Input: part model. Units: mm. Frame: model coordinates. A direction names the side the tool comes from. Give positions to 0.01 mm unless a question says otherwise; leave off trailing zeros. Write each loop counter-clockwise with the first axis right and the second up, starting at its lowest first coordinate (ties: lowest second). Pieces come first, ordered by that corner, then holes. Notation, with made-up numbers: (88.5, 43.5) -> (126.5, 43.5) arc R35 ccw to (126.5, 75.5) -> close; hole circle Ø11 at (22, 50.25). An arc over 180 degrees is marked (long way). Return JSON: item names as keys, results as strings. Group by question number.
Item 1: Section C-C, the plane y = 13. Return loops of the section in (x, z) (3 decimals), then the cut area to 3 significant figures.
Item 2: Section B-B, the plane x = 0. Return loops of the section in (y, z) (3 decimals).
Item 3: Mould query, pull axis Y, two halves, no side actions, for faces 3 (the face through (38.1, -1.5, 3.9)), 4 (the face through (27.746, 10.498, -23.835)), 5 (the face through (-1, -3.175, 7)). Classes: released by +Y, released by -Y, zero draft, split by the parting line, or undercut.
Item 4: Section A-A, the plane x = 25.4. Return loops of the section in (y, z) (3 decimals).
Item 5: Set-up query: faces 1 (the face through (-27.332, -1.565, 27.025)), 2 (the face through (-1, 0, 8)). Return all of +Z, -Z, +X, -X, +Y, -Y with unobstructed straight access to the full face (end or side cutting, diameter ignored); none if empty.
Item 6: Section D-D, the plane z = 6. Return loops of the section in (x, y) (3 decimals), then the cut area to 3 significant figures.
Item 7: Pin query (flat end, axial travel): P1, Ø6, axis at x = 0, z = -3.175, coming from the -Y side; P2, Ø6, axis at x = -21.5, z = 19.5, coming from the +Y side. Return the tip coordinate at first contact, or that it passes through.
Item 8: Line query: line 1 (Z direction, x = 19, y = -1); line 2 (Y direction, x = 25.4, z = -23.85) (3 decimals); line 3 (Y direction, x = -27.5, z = 11) (3 decimals). Output: solid intervals per line, ascending. Write a range as [from, to].
from build123d import *

# Parameters (mm, degrees)
F0_W     = 76.2
F0_H     = 63.5
F0_R     = 1.5875
F0_R_2   = 3.81
F1_DEPTH = 3.175
F3_W     = 76.2
F3_H     = 19.05
F3_R     = 2.54
F4_DEPTH = 3.175
F5_R     = 1.27


with BuildPart() as f1:
    # F0 (on Front) → F1 (new body)
    with BuildSketch(Plane.XZ):
        with Locations((0, 6.35)):
            Rectangle(F0_W, F0_H)
        with Locations((-26.9875, -3.175)):
            Circle(F0_R, mode=Mode.SUBTRACT)
        with Locations((-19.05, -3.175)):
            Circle(F0_R_2, mode=Mode.SUBTRACT)
        with Locations((-7.9375, -3.175)):
            Circle(F0_R, mode=Mode.SUBTRACT)
        with Locations((0, -3.175)):
            Circle(F0_R_2, mode=Mode.SUBTRACT)
        with Locations((11.1125, -3.175)):
            Circle(F0_R, mode=Mode.SUBTRACT)
        with Locations((19.05, -3.175)):
            Circle(F0_R_2, mode=Mode.SUBTRACT)
        with Locations((-26.9875, 28.575)):
            Circle(F0_R, mode=Mode.SUBTRACT)
        with Locations((-19.05, 28.575)):
            Circle(F0_R_2, mode=Mode.SUBTRACT)
        with Locations((-7.9375, 28.575)):
            Circle(F0_R, mode=Mode.SUBTRACT)
        with Locations((0, 28.575)):
            Circle(F0_R_2, mode=Mode.SUBTRACT)
        with Locations((11.1125, 28.575)):
            Circle(F0_R, mode=Mode.SUBTRACT)
        with Locations((19.05, 28.575)):
            Circle(F0_R_2, mode=Mode.SUBTRACT)
    extrude(amount=F1_DEPTH)

    # F3 (on face) → F4 (join)
    with BuildSketch(Plane(origin=(0, 0, -25.4), x_dir=(1, 0, 0), z_dir=(0, 0, -1))):
        with Locations((0, -9.525)):
            Rectangle(F3_W, F3_H)
        with Locations((-25.4, -9.525)):
            Circle(F3_R, mode=Mode.SUBTRACT)
        with Locations((25.4, -9.525)):
            Circle(F3_R, mode=Mode.SUBTRACT)
    extrude(amount=-F4_DEPTH)

    # F5
    f5_edges = [f1.edges().sort_by_distance(p)[0] for p in [
        (38.1, -3.175, 6.35),
        (38.1, 0, 7.9375),
        (-38.1, -3.175, 6.35),
        (-38.1, 0, 7.9375),
        (0, 0, 38.1),
        (0, -3.175, 38.1),
        (0, 0, -22.225),
        (0, 19.05, -22.225),
        (38.1, 7.9375, -25.4),
        (38.1, -1.5875, 38.1),
        (38.1, 9.525, -22.225),
        (38.1, 19.05, -23.8125),
        (0, 19.05, -25.4),
        (-38.1, 7.9375, -25.4),
        (0, -3.175, -25.4),
        (-38.1, 9.525, -22.225),
    ]]
    fillet(f5_edges, radius=F5_R)


solid = f1.part
Answer below:
{
 "1": {"outline": "(-38.1, -24.13) arc R1.27 ccw to (-36.83, -25.4) -> (36.83, -25.4) arc R1.27 ccw to (38.1, -24.13) -> (38.1, -23.495) arc R1.27 ccw to (36.83, -22.225) -> (-36.83, -22.225) arc R1.27 ccw to (-38.1, -23.495) -> close", "area": "241 mm2"},
 "2": {"outline": "(-3.175, -24.13) arc R1.27 ccw to (-1.905, -25.4) -> (17.78, -25.4) arc R1.27 ccw to (19.05, -24.13) -> (19.05, -23.495) arc R1.27 ccw to (17.78, -22.225) -> (1.27, -22.225) arc R1.27 cw to (0, -20.955) -> (0, -6.985) -> (-3.175, -6.985) -> close; (-3.175, 0.635) -> (0, 0.635) -> (0, 24.765) -> (-3.175, 24.765) -> close; (-3.175, 32.385) -> (0, 32.385) -> (0, 36.83) arc R1.27 ccw to (-1.27, 38.1) -> (-1.905, 38.1) arc R1.27 ccw to (-3.175, 36.83) -> close"},
 "3": {"face 3": "zero draft", "face 4": "undercut", "face 5": "released by -Y"},
 "4": {"outline": "(-3.175, -24.13) arc R1.27 ccw to (-1.905, -25.4) -> (6.985, -25.4) -> (6.985, -22.225) -> (1.27, -22.225) arc R1.27 cw to (0, -20.955) -> (0, 36.83) arc R1.27 ccw to (-1.27, 38.1) -> (-1.905, 38.1) arc R1.27 ccw to (-3.175, 36.83) -> close; (12.065, -25.4) -> (17.78, -25.4) arc R1.27 ccw to (19.05, -24.13) -> (19.05, -23.495) arc R1.27 ccw to (17.78, -22.225) -> (12.065, -22.225) -> close"},
 "5": {"face 1": "+Y, -Y", "face 2": "+Z, +X, -X, +Y"},
 "6": {"outline": "(-38.1, -1.905) arc R1.27 ccw to (-36.83, -3.175) -> (36.83, -3.175) arc R1.27 ccw to (38.1, -1.905) -> (38.1, -1.27) arc R1.27 ccw to (36.83, 0) -> (-36.83, 0) arc R1.27 ccw to (-38.1, -1.27) -> close", "area": "241 mm2"},
 "7": {"P1": "passes through", "P2": "stops at y = 0"},
 "8": {"line 1": "z = [-25.4, -6.98], [0.63, 24.77], [32.38, 38.07]", "line 2": "y = [-3.175, 6.985], [12.065, 19.05]", "line 3": "y = [-3.175, 0]"}
}
